Source: three-view drawing plus pictorial views. Frame: mm from the lowest corner of the part. A direction names the side the tool comes from. Give positions to 0.01 mm unless a question says otherwise; leave off trailing zeros. Order: outer loops, then holes, each group sorted by start corner. A loop starts at its lowest first (then second) coordinate and runs counter-clockwise, first axis right, second up. Notation, with made-up numbers: (31.25, 30) - (87.25, 30) arc R12 cw to (87.25, 51) - close; hole circle Ø3 at (-19, 38.5). An arc over 180 degrees is marked (long way). Use one line per item in the form item = value.
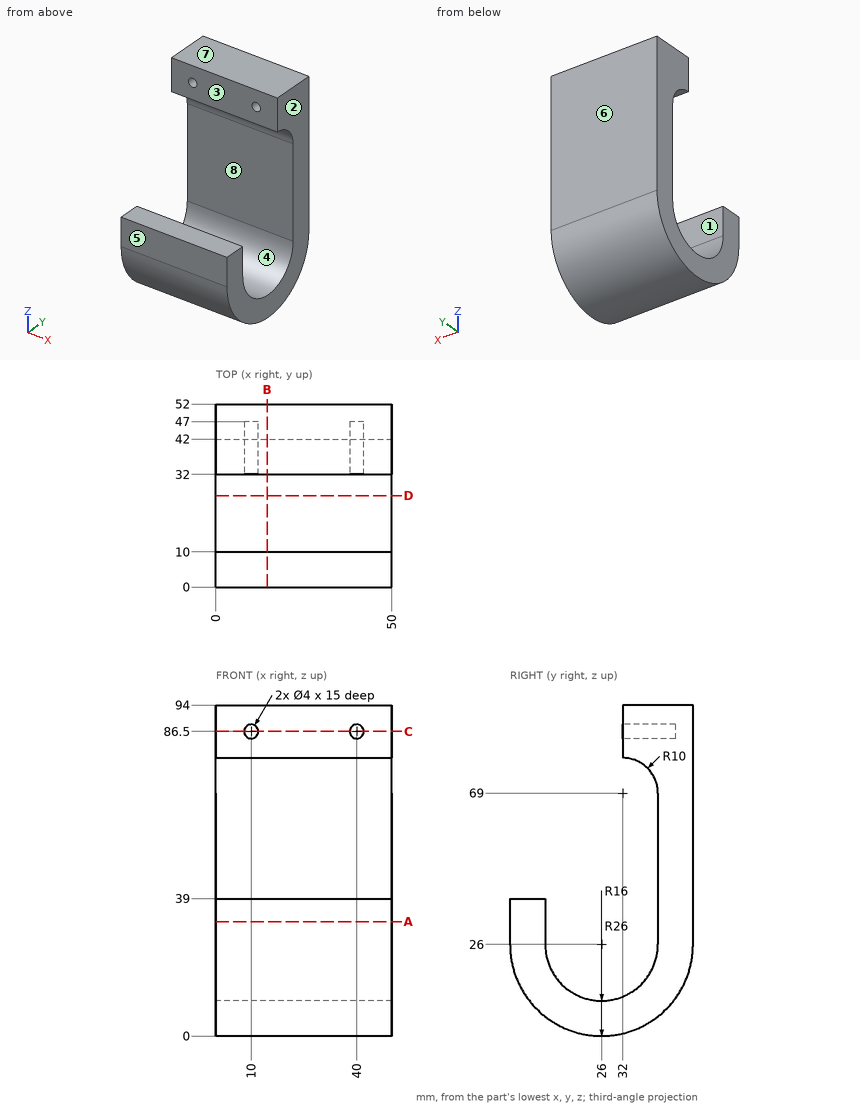
(1) Pull-direction query (Z, two-part tool) for the marked faces 6, 7 and 8; classes: released by +Z, released by -Z, zero draft, split by the parting line, or undercut.
Computed values:
face_6 = zero draft
face_7 = released by +Z
face_8 = undercut
(2) Cut plane A-A on z = 32.5. Output: boundary loops of the cut face in (x, y), plus the area to 3 significant figures.
Computed values:
outline = (0, 0) - (50, 0) - (50, 10) - (0, 10) - close; (0, 42) - (50, 42) - (50, 52) - (0, 52) - close
area = 1,000 mm²
(3) Cut plane C-C on z = 86.5. Output: boundary loops of the cut face in (x, y), plus the area to 3 significant figures.
Computed values:
outline = (0, 32) - (8, 32) - (8, 47) - (12, 47) - (12, 32) - (38, 32) - (38, 47) - (42, 47) - (42, 32) - (50, 32) - (50, 52) - (0, 52) - close
area = 880 mm²
(4) Reachability of the marked faces 1, 2, 3, 4 and 5 from +Z, -Z, +X, -X, +Y, -Y: full face, straight path, thin tool, end or side. Return the list, or none.
Computed values:
face_1 = +Z, +X, -X
face_2 = +Z, -Z, +X, +Y, -Y
face_3 = +Z, +X, -X, -Y
face_4 = +X, -X
face_5 = +Z, -Z, +X, -X, -Y
(5) Ray query, line 1 along Y through (x, z) = (41, 26); line 2 along X through (y, z) = (43, 86); line 3 along Z through (x, y) = (10, 39.75). Return the intervals inside material, ascending.
Computed values:
line_1 = 0 to 10, 42 to 52
line_2 = 0 to 8.06, 11.94 to 38.06, 41.94 to 50
line_3 = 3.93 to 17.82, 75.32 to 84.5, 88.5 to 94
(6) Cut plane B-B on x = 14.5. Output: boundary loops of the cut face in (y, z).
Computed values:
outline = (0, 26) arc R26 ccw to (52, 26) - (52, 94) - (32, 94) - (32, 79) arc R10 cw to (42, 69) - (42, 26) arc R16 cw to (10, 26) - (10, 39) - (0, 39) - close
(7) Cut plane D-D on y = 26. Output: boundary loops of the cut face in (x, z), plus the area to 3 significant figures.
Computed values:
outline = (0, 0) - (50, 0) - (50, 10) - (0, 10) - close
area = 500 mm²
(8) Contact query for flat-ended pins moving along their axis: pin 1 Ø2 at (x, y) = (32.5, 45.5) entering from -Z; pin 2 Ø1 at (x, z) = (11, 19) entering from +Y; pin 3 Ø3 at (x, z) = (10.5, 85.5) entering from -Y. Output: stop coordinate, or through.
Computed values:
pin_1 = 7.73
pin_2 = 51.17
pin_3 = 32
